```python
from build123d import *

# Parameters (mm, degrees)
F1_DEPTH = 825


with BuildPart() as f1:
    # F0 (on Right) → F1 (new body, symmetric)
    with BuildSketch(Plane.YZ):
        Polygon((70, 60), (70, 70), (-70, 70), (-70, 60), (-4, 60), (-4, -60), (-70, -60), (-70, -70), (70, -70), (70, -60), (4, -60), (4, 60), align=None)
    extrude(amount=F1_DEPTH, both=True)


solid = f1.part
```
Could you check a few things on this model? Use its own coordinates, in mm. A direction names the side the tool comes from. Coordinates: 2 decimals unless noted, no trailing zeros. Order: outer loops, then holes, each group sorted by start corner. A loop starts at its lowest first (then second) coordinate and runs counter-clockwise, first axis right, second up. Notation, with made-up numbers: M 10,0 L 28,0 A24 cw 28,19 Z; hole C -36,77 d1. An arc over 180 degrees is marked long. Use a Markdown table: item, result. Add a question column.
Q1. I want a section at B-B on x = 658. List the corners of the cut face in (y, z) for me, then the cut area to 3 significant figures.
Q2. I'm going to push a flat-ended pin straight in: pin 1 (8 mm diameter, centred on x = 184, z = -29, fed in from -Y). Where does the tip first touch, or does it pass through?
Q3. I want a section at C-C on z = -0.5. List the corners of the cut face in (x, y) for me.
Q4. I want a section at A-A on y = 54. List the corners of the cut face in (x, z) for me, then the cut area to 3 significant figures.
Q5. Which directions (+Z, -Z, +X, -X, +Y, -Y) give clear straight access to the entire face, cutting with the end or side of a thin tool? Please do faces 5 (the flat face through (12, 37, -60)), 6 (the flat face through (-825, 0, -5)), 7 (the flat face through (12, -37, 60)).
Q6. We'd pull the mould along Z, two halves only. Please class faces 1 (the flat face through (825, 0, -5)), 2 (the flat face through (12, 1, 70)), 3 (the flat face through (12, 4, -1)), 4 (the flat face through (12, -1, -70)): pulls with the +Z half, pulls with the -Z half, needs draft (parallel to the pull), parting line crosses it, or undercut.
Q7. If I drill on L1, parallel to Z at x = 622, y = 37; L2, parallel to Y at x = 678.5, z = 17.5, over which ranges is the centre line in solid material (lowest first)?
Checked values:
| question | item | result |
|---|---|---|
| 1 | outline | M -70,-70 L 70,-70 L 70,-60 L 4,-60 L 4,60 L 70,60 L 70,70 L -70,70 L -70,60 L -4,60 L -4,-60 L -70,-60 Z |
| 1 | area | 3,760 mm² |
| 2 | pin 1 | y = -4 |
| 3 | outline | M -825,-4 L 825,-4 L 825,4 L -825,4 Z |
| 4 | outline | M -825,-70 L 825,-70 L 825,-60 L -825,-60 Z; M -825,60 L 825,60 L 825,70 L -825,70 Z |
| 4 | area | 33,000 mm² |
| 5 | face 5 | +X, -X, +Y |
| 5 | face 6 | +Z, -Z, -X, +Y, -Y |
| 5 | face 7 | +X, -X, -Y |
| 6 | face 1 | needs draft |
| 6 | face 2 | pulls with the +Z half |
| 6 | face 3 | undercut |
| 6 | face 4 | pulls with the -Z half |
| 7 | L1 | -70 to -60, 60 to 70 |
| 7 | L2 | -4 to 4 |
